Here's the drawing with two shaded views (mm, measured from the low corner). I have some questions. A direction names the side the tool comes from. Round coordinates to 2 decimals unless told otherwise and drop trailing zeros. Write each loop counter-clockwise with the first axis right and the second up, starting at its lowest first coordinate (ties: lowest second). Pieces come first, ordered by that corner, then holes. Notation, with made-up numbers: (25.5, 61.5) -> (81.5, 61.5) arc R18 ccw to (81.5, 87.5) -> close; hole circle Ø4 at (-18.5, 34). An arc over 180 degrees is marked (long way). Use CSV: the item, a comma, the result in double quotes.
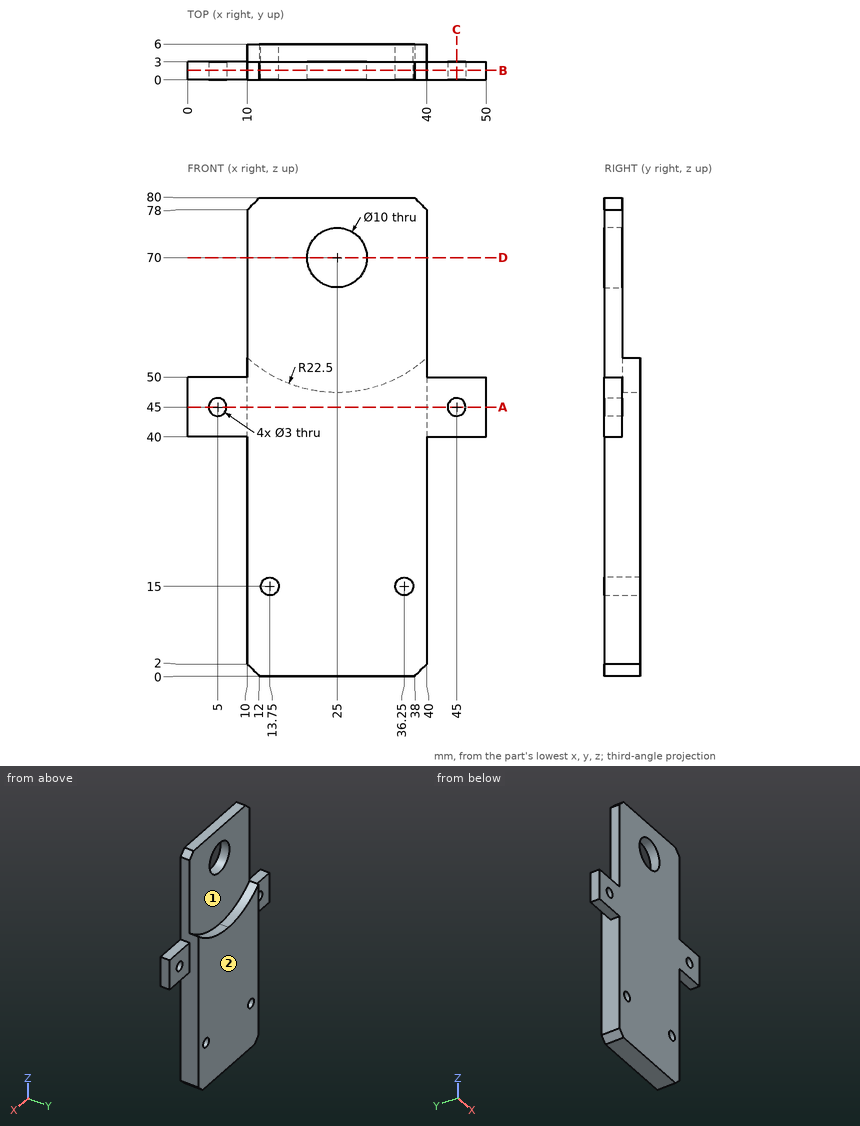
Q1. On a 3-axis mill with a long thin cutter (end or side, diameter ignored), from which of +Z, -Z, +X, -X, +Y, -Y can I reach the whole of each face in a straight line? I mean the marked faces 1 and 2. Say none if no direction works.
Resolved:
face 1,"+Z, +Y"
face 2,"+Z, -Z, +X, -X, +Y"
Q2. Suppose I cut it at D-D (z = 70). Write out the boundary of the cut face in (x, y), and give its area (3 significant figures).
Resolved:
outline,"(10, 0) -> (20, 0) -> (20, 3) -> (10, 3) -> close; (30, 0) -> (40, 0) -> (40, 3) -> (30, 3) -> close"
area,"60.0 mm^2"
Q3. Suppose I cut it at A-A (z = 45). Write out the boundary of the cut face in (x, y), and give its area (3 significant figures).
Resolved:
outline,"(0, 0) -> (3.5, 0) -> (3.5, 3) -> (0, 3) -> close; (6.5, 0) -> (43.5, 0) -> (43.5, 3) -> (40, 3) -> (40, 6) -> (10, 6) -> (10, 3) -> (6.5, 3) -> close; (46.5, 0) -> (50, 0) -> (50, 3) -> (46.5, 3) -> close"
area,"222 mm^2"
Q4. Suppose I cut it at C-C (x = 45). Write out the boundary of the cut face in (y, z).
Resolved:
outline,"(0, 40) -> (3, 40) -> (3, 43.5) -> (0, 43.5) -> close; (0, 46.5) -> (3, 46.5) -> (3, 50) -> (0, 50) -> close"
Q5. Will these pins go through, and if not, where does the flat tip stop? P1, Ø16, axis at x = 25, z = 70, coming from the +Y side; P2, Ø2.5, axis at x = 5, z = 45, coming from the +Y side; P3, Ø3, axis at y = 1, z = 19.5, coming from the -X side; P4, Ø0.9, axis at x = 44.5, y = 1.5, coming from the -Z side.
Resolved:
P1,"stops at y = 3"
P2,"passes through"
P3,"stops at x = 10"
P4,"stops at z = 40"
Q6. Suppose I cut it at B-B (y = 1.6). Write out the boundary of the cut face in (x, z).
Resolved:
outline,"(0, 40) -> (10, 40) -> (10, 2) -> (12, 0) -> (38, 0) -> (40, 2) -> (40, 40) -> (50, 40) -> (50, 50) -> (40, 50) -> (40, 78) -> (38, 80) -> (12, 80) -> (10, 78) -> (10, 50) -> (0, 50) -> close; hole circle Ø3 at (5, 45); hole circle Ø3 at (13.75, 15); hole circle Ø10 at (25, 70); hole circle Ø3 at (36.25, 15); hole circle Ø3 at (45, 45)"
Q7. Please list where these lines run through material, in increasing order: probe 1 along X at (y, z) = (4.55, 15); probe 2 along X at (y, z) = (0.3, 16); probe 3 along X at (y, z) = (1.05, 70).
Resolved:
probe 1,"x = 10 to 12.25, 15.25 to 34.75, 37.75 to 40"
probe 2,"x = 10 to 12.63, 14.87 to 35.13, 37.37 to 40"
probe 3,"x = 10 to 20, 30 to 40"
